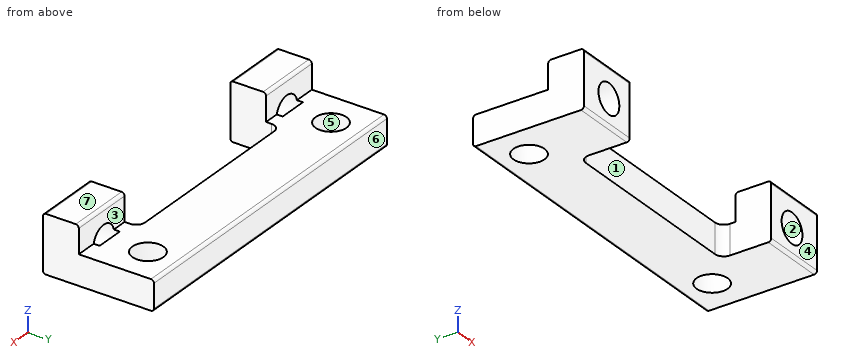
from build123d import *

# Parameters (mm, degrees)
SKETCH_1_W               = 28
SKETCH_1_H               = 9.3
EXTRUDE_1_DEPTH          = 4.8
SKETCH_2_W               = 28
SKETCH_2_H               = 6.3
CUT_EXTRUDE_1_DEPTH      = 2.3
SKETCH_4_W               = 17
SKETCH_4_H               = 4.2
CUT_EXTRUDE_2_DEPTH      = 1
CUT_EXTRUDE_2_DEPTH_BACK = 5.8
SKETCH_5_R               = 1.3
CUT_EXTRUDE_3_DEPTH      = 3.5
FILLET_1_R               = 0.75
SKETCH_6_R               = 1.25
CUT_EXTRUDE_4_DEPTH      = 3.5
FILLET_2_R               = 0.25


with BuildPart() as part:
    # 스케치1 → 보스-돌출1 (new body)
    with BuildSketch(Plane.XY):
        with Locations((14, 4.65)):
            Rectangle(SKETCH_1_W, SKETCH_1_H)
    extrude(amount=EXTRUDE_1_DEPTH)

    # 스케치2 → 컷-돌출1 (cut)
    with BuildSketch(Plane.XY.offset(4.8)):
        with Locations((14, 6.15)):
            Rectangle(SKETCH_2_W, SKETCH_2_H)
    extrude(amount=-CUT_EXTRUDE_1_DEPTH, mode=Mode.SUBTRACT)

    # 스케치4 → 컷-돌출2 (cut, two sides)
    with BuildSketch(Plane.XY.offset(4.8)) as cut_extrude_2_sk:
        with Locations((14, 2.1)):
            Rectangle(SKETCH_4_W, SKETCH_4_H)
    extrude(amount=CUT_EXTRUDE_2_DEPTH, mode=Mode.SUBTRACT)
    extrude(cut_extrude_2_sk.sketch, amount=-CUT_EXTRUDE_2_DEPTH_BACK, mode=Mode.SUBTRACT)

    # 스케치5 → 컷-돌출3 (cut, through all)
    with BuildSketch(Plane.XY.offset(2.5)):
        with Locations((3, 6.7)):
            Circle(SKETCH_5_R)
        with Locations((25, 6.7)):
            Circle(SKETCH_5_R)
    extrude(amount=-CUT_EXTRUDE_3_DEPTH, mode=Mode.SUBTRACT)

    # 필렛1
    fillet_1_edges = [part.edges().sort_by_distance(p)[0] for p in [
        (5.5, 4.2, 1.25),
        (22.5, 4.2, 1.25),
    ]]
    fillet(fillet_1_edges, radius=FILLET_1_R)

    # 스케치6 → 컷-돌출4 (cut)
    with BuildSketch(Plane.XZ):
        with Locations((3, 2.2)):
            Circle(SKETCH_6_R)
        with Locations((25, 2.2)):
            Circle(SKETCH_6_R)
    extrude(amount=-CUT_EXTRUDE_4_DEPTH, mode=Mode.SUBTRACT)

    # 필렛2
    fillet_2_edges = [part.edges().sort_by_distance(p)[0] for p in [
        (14, 9.3, 2.5),
        (2.75, 3, 4.8),
        (25.25, 3, 4.8),
        (25.25, 0, 0),
        (25.25, 0, 4.8),
        (14, 9.3, 0),
        (2.75, 0, 0),
        (2.75, 0, 4.8),
    ]]
    fillet(fillet_2_edges, radius=FILLET_2_R)


solid = part.part
Work out the finished part from the listing and answer in its coordinate system (mm). Face numbers are marked on the shaded views. A direction names the side the tool comes from. Round coordinates to 2 decimals unless told otherwise and drop trailing zeros. Loops run counter-clockwise (first coordinate to the right, second up) from the corner with the lowest first, then second, coordinate; pieces in that order, holes last. Notation, with made-up numbers: (-6.75, -26.5) - (35.25, -26.5) arc R22 ccw to (35.25, 2.5) - close; hole circle Ø10 at (-37.5, 60). An arc over 180 degrees is marked (long way). Use one line per item in the form item = value. Start each with the question number.
(1) Which of the six approach directions +Z, -Z, +X, -X, +Y, -Y give full straight-line access (tool end or side, diameter ignored) to the marked faces 1, 2 and 3?
(2) Find section A-A on y = 1.25. Determine the outline of the cut face in (x, z), and give its area (3 significant figures).
(3) Find section D-D on y = 6.7. Determine the outline of the cut face in (x, z), and give its area (3 significant figures).
(4) Consider line 1 (X direction, y = 0.75, z = 2.2); line 2 (Z direction, x = 25, y = 2.2); line 3 (X direction, y = 6.5, z = 1.6). Determine where each line is inside the solid, lowest interval first.
(5) Determine the mould class of the marked faces 4, 5, 6 and 7 for opening direction Y: +Y half, -Y half, draft (parallel to the pull), parting line (faces both ways), or undercut.
(6) Find section B-B on x = 3. Determine the outline of the cut face in (y, z).
(7) Flat-ended cylindrical pins translate along their axes: P1, Ø0.8, axis at x = 10.5, z = 1, coming from the -Y side; P2, Ø1.2, axis at x = 24.5, z = 2, coming from the -Y side; P3, Ø2.5, axis at x = 24.5, z = 4, coming from the +Y side. Find the tip coordinate at first contact, or state that the pin passes through.
(8) Find section C-C on z = 3.2. Determine the outline of the cut face in (x, y).
Answer list:
q1.face_1 = +Z, -Z, -Y
q1.face_2 = -Y
q1.face_3 = +Z, +X, -X, +Y
q2.outline = (0, 0) - (5.5, 0) - (5.5, 4.8) - (0, 4.8) - close; (22.5, 0) - (28, 0) - (28, 4.8) - (22.5, 4.8) - close; hole circle Ø2.5 at (3, 2.2); hole circle Ø2.5 at (25, 2.2)
q2.area = 43.0 mm^2
q3.outline = (0, 0) - (1.7, 0) - (1.7, 2.5) - (0, 2.5) - close; (4.3, 0) - (23.7, 0) - (23.7, 2.5) - (4.3, 2.5) - close; (26.3, 0) - (28, 0) - (28, 2.5) - (26.3, 2.5) - close
q3.area = 57.0 mm^2
q4.line_1 = 0 to 1.75, 4.25 to 5.5, 22.5 to 23.75, 26.25 to 28
q4.line_2 = 0 to 0.95, 3.45 to 4.8
q4.line_3 = 0 to 1.72, 4.28 to 23.72, 26.28 to 28
q5.face_4 = -Y half
q5.face_5 = undercut
q5.face_6 = +Y half
q5.face_7 = draft
q6.outline = (0, 0.25) arc R0.25 ccw to (0.25, 0) - (5.4, 0) - (5.4, 2.5) - (3.5, 2.5) - (3.5, 0.95) - (0, 0.95) - close; (0, 3.45) - (3, 3.45) - (3, 4.55) arc R0.25 ccw to (2.75, 4.8) - (0.25, 4.8) arc R0.25 ccw to (0, 4.55) - close; (8, 0) - (9.05, 0) arc R0.25 ccw to (9.3, 0.25) - (9.3, 2.25) arc R0.25 ccw to (9.05, 2.5) - (8, 2.5) - close
q7.P1 = 4.2
q7.P2 = 3.5
q7.P3 = 3
q8.outline = (0, 0) - (2.25, 0) - (2.25, 3) - (0, 3) - close; (3.75, 0) - (5.5, 0) - (5.5, 3) - (3.75, 3) - close; (22.5, 0) - (24.25, 0) - (24.25, 3) - (22.5, 3) - close; (25.75, 0) - (28, 0) - (28, 3) - (25.75, 3) - close
